Part model, mm, in its own coordinate system. Face numbers are marked on the shaded views. A direction names the side the tool comes from. Give positions to 0.01 mm unless a question says otherwise; leave off trailing zeros. Loops run counter-clockwise (first coordinate to the right, second up) from the corner with the lowest first, then second, coordinate; pieces in that order, holes last. Notation, with made-up numbers: M 69,26 L 78,26 A16 ccw 78,44 Z; hole C 8.25,63.25 d6. An arc over 180 degrees is marked long. Answer in a Markdown table with one row per item.
from build123d import *

# Parameters (mm, degrees)
F1_DEPTH = 300
F3_D     = 50
F5_D     = 50
F7_D     = 50


with BuildPart() as f1:
    # F0 (on Front) → F1 (new body)
    with BuildSketch(Plane.XZ):
        Polygon((0, 221.130219), (0, 0), (900, 0), (900, 652.334173), (600, 652.334173), (600, 437.837817), (300, 437.837817), (300, 221.130219), align=None)
    extrude(amount=F1_DEPTH)

    # F3 (through all)
    with Locations(Plane.XY.offset(437.837817)):
        with Locations((450, -150)):
            Hole(F3_D / 2)

    # F5 (through all)
    with Locations(Plane.XY.offset(221.130219)):
        with Locations((150, -150)):
            Hole(F5_D / 2)

    # F7 (through all)
    with Locations(Plane.XY.offset(652.334173)):
        with Locations((750, -150)):
            Hole(F7_D / 2)


solid = f1.part
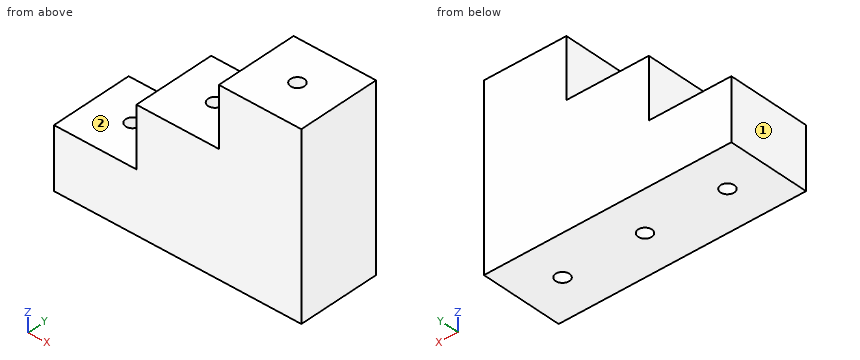
(1) Which spindle directions (+Z, -Z, +X, -X, +Y, -Y) get a long thin tool onto all of the face, cutting with end or side? Do the marked faces 1 and 2. Say none if no direction does.
Recorded:
| item | result |
|---|---|
| face 1 | +Z, -Z, -X, +Y, -Y |
| face 2 | +Z, -X, +Y, -Y |
(2) Saw through at A-A (x = 750). Write the cut outline in (y, z), plus the area to 3 significant figures.
Recorded:
| item | result |
|---|---|
| outline | M -300,0 L -175,0 L -175,652.33 L -300,652.33 Z; M -125,0 L 0,0 L 0,652.33 L -125,652.33 Z |
| area | 163,000 mm^2 |
(3) Pin check, flat tip, straight feed: pin 1 Ø12 at (x, y) = (183, -51) entering from +Z. Stop position of the tip, or through.
Recorded:
| item | result |
|---|---|
| pin 1 | stops at z = 221.13 |
(4) Saw through at B-B (y = -150). Write the cut outline in (x, z), plus the area to 3 significant figures.
Recorded:
| item | result |
|---|---|
| outline | M 0,0 L 125,0 L 125,221.13 L 0,221.13 Z; M 175,0 L 425,0 L 425,437.84 L 300,437.84 L 300,221.13 L 175,221.13 Z; M 475,0 L 725,0 L 725,652.33 L 600,652.33 L 600,437.84 L 475,437.84 Z; M 775,0 L 900,0 L 900,652.33 L 775,652.33 Z |
| area | 328,000 mm^2 |
(5) Drill centre lines: line 1 along X through (y, z) = (-147, 90.5); line 2 along Y through (x, z) = (750, 298); line 3 along Z through (x, y) = (597, -267.5). Where is each one in solid material? Low to high.
Recorded:
| item | result |
|---|---|
| line 1 | x = 0 to 125.18, 174.82 to 425.18, 474.82 to 725.18, 774.82 to 900 |
| line 2 | y = -300 to -175, -125 to 0 |
| line 3 | z = 0 to 437.84 |
(6) Saw through at D-D (y = -259). Write the cut outline in (x, z), plus the area to 3 significant figures.
Recorded:
| item | result |
|---|---|
| outline | M 0,0 L 900,0 L 900,652.33 L 600,652.33 L 600,437.84 L 300,437.84 L 300,221.13 L 0,221.13 Z |
| area | 393,000 mm^2 |
(7) Saw through at C-C (z = 92). Write the cut outline in (x, y), plus the area to 3 significant figures.
Recorded:
| item | result |
|---|---|
| outline | M 0,-300 L 900,-300 L 900,0 L 0,0 Z; hole C 150,-150 d50; hole C 450,-150 d50; hole C 750,-150 d50 |
| area | 264,000 mm^2 |
